Could you check a few things on this model? Use its own coordinates, in mm. Coordinates: 2 decimals unless noted, no trailing zeros. Loops run counter-clockwise (first coordinate to the right, second up) from the corner with the lowest first, then second, coordinate; pieces in that order, holes last. Notation, with made-up numbers: (2, 50.5) - (43, 50.5) arc R22 cw to (43, 87.5) - close; hole circle Ø2 at (15.25, 22). An arc over 180 degrees is marked (long way). One line per item, written item: value. Start each with the question number.
(1) If we section it at B-B on x = -54.5: Write out the boundary of the cut face in (y, z).
(2) If I drill on line 1 along Z through (x, y) = (31, -18); line 2 along Z through (x, y) = (37, -36), over which ranges is the centre line in solid material (lowest first)? Write a range as from..to.
(3) If we mould it in two halves opening along Z, with no side actions, what happens to faces 1 (the face through (-43.2, 0, -13.6)), 2 (the face through (-22.572, -34.51, -6.587)), 3 (the face through (43.35, -34.51, 14.48)), 4 (the face through (42.047, -34.51, 13.997))? For each: pulls with the +Z half, pulls with the -Z half, needs draft (parallel to the pull), parting line crosses it, or undercut.
(4) I'm going to push flat-ended pins straight in: P1, Ø1, axis at x = -61, y = -61.5, coming from the +Z side; P2, Ø12, axis at x = 13.5, y = -12.5, coming from the +Z side; P3, Ø2, axis at x = -10.5, y = -25.5, coming from the -Z side. Where does each tip first touch, or does it pass through?
(5) If we section it at A-A on y = -17: Write out the boundary of the cut face in (x, z), then the cut area to 3 significant figures.
(6) If we section it at C-C on z = -19.5: Write out the boundary of the cut face in (x, y).
```python
from build123d import *

# Parameters (mm, degrees)
F1_DEPTH = 70


with BuildPart() as f1:
    # F0 (on Front) → F1 (new body)
    with BuildSketch(Plane.XZ):
        with BuildLine():
            ThreePointArc((38.684679, 14.981631), (42.07904, 13.954538), (42.122397, 10.408452))
            Line((42.122397, 10.408452), (43.112431, 9.482922))
            ThreePointArc((43.112431, 9.482922), (43.308922, 14.546989), (38.574926, 16.356039))
            Line((38.574926, 16.356039), (37.950457, 16.139805))
            Line((37.950457, 16.139805), (-82.800867, -25.672631))
            Line((-82.800867, -25.672631), (-82.136644, -27.559111))
            Line((-82.136644, -27.559111), (38.684679, 14.981631))
        make_face()
    extrude(amount=F1_DEPTH)


solid = f1.part
```
Values:
1. outline: (-70, -17.83) - (0, -17.83) - (0, -15.87) - (-70, -15.87) - close
2. line 1: z = 12.28..13.73
2. line 2: z = 14.39..15.81
3. face 1: needs draft
3. face 2: pulls with the -Z half
3. face 3: parting line crosses it
3. face 4: undercut
4. P1: stops at z = -17.95
4. P2: stops at z = 9.75
4. P3: stops at z = -2.69
5. outline: (-82.8, -25.67) - (-82.14, -27.56) - (38.68, 14.98) arc R3 cw to (42.12, 10.41) - (43.11, 9.48) arc R4.35 ccw to (38.57, 16.36) - (37.95, 16.14) - close
5. area: 226 mm2
6. outline: (-64.97, -70) - (-59.25, -70) - (-59.25, 0) - (-64.97, 0) - close
